The model under review builds one solid part; all positions refer to its coordinate system, in mm. A direction names the side the tool comes from. Give positions to 0.01 mm unless a question says otherwise; leave off trailing zeros. Order: outer loops, then holes, each group sorted by start corner. A loop starts at its lowest first (then second) coordinate and runs counter-clockwise, first axis right, second up. Notation, with made-up numbers: (64.5, 69.25) - (81.5, 69.25) arc R18 ccw to (81.5, 99.25) - close; hole circle Ø2 at (84.25, -23). An arc over 180 degrees is marked (long way). Write item = value, one per line. Start each with the question number.
1. Machinability: for faces 5 (the cylindrical face through (-17, -1, 15)), 6 (the cylindrical face through (-33.56, -29.22, 6.85)), 7 (the cylindrical face through (-17, -15, 24)), 8 (the flat face through (1, -15, -21.822)), 9 (the cylindrical face through (-16.5, -29.22, 15.24)), which of the approach directions +Z, -Z, +X, -X, +Y, -Y give a long, thin tool a straight path to every point of the face, cutting with its end or side? Answer none if there is none.
2. Mouldability with a two-part tool opening along X and no side actions: class faces 1 (the cylindrical face through (16, -15, 23)), 2 (the cylindrical face through (59, -1, 23)), 3 (the flat face through (-100, -15, 0)), 4 (the flat face through (15, -15, 15)) as pulls with the +X half, pulls with the -X half, needs draft (parallel to the pull), parting line crosses it, or undercut.
3. We need section C-C, the plane z = 22.5. Give the boundary of the cut face in (x, y) (3 decimals), and give its area (3 significant figures).
4. We need section B-B, the plane z = -19.5. Give the boundary of the cut face in (x, y).
5. Wall thickness on probe 1 along X at (y, z) = (-16, -12); probe 2 along Y at (x, z) = (32.6, 16.5) (3 decimals); probe 3 along X at (y, z) = (-18, 15.5): over which ranges is each line inside the solid? List them lowest first.
6. We need section A-A, the plane x = 32.6. Give the boundary of the cut face in (y, z) (3 decimals).
7. We need section D-D, the plane y = -21. Give the boundary of the cut face in (x, z), and give its area (3 significant figures).
8. For P1, Ø8, axis at x = -10.5, y = -11, coming from the +Z side, flat-tipped, find the tip position at first contact; note if it passes through.
from build123d import *

# Parameters (mm, degrees)
F1_DEPTH  = 30.65
F2_R      = 5
F3_R      = 5
F4_R      = 5
F5_R      = 5
F6_R      = 5
F7_R      = 5
F8_R      = 5
F9_R      = 5
F10_R     = 3
F11_DEPTH = 20


with BuildPart() as f1:
    # F0 (on Front) → F1 (new body)
    with BuildSketch(Plane.XZ):
        Polygon((-100, 25), (-100, -25), (100, -25), (100, 25), (15, 25), (15, 5.35), (47.5, 5.35), (47.5, -7.066266), (47.5, -21.822188), (0, -21.822188), (-47.5, -21.822188), (-47.5, -7.066266), (-47.5, 5.35), (-15, 5.35), (-15, 25), align=None)
    extrude(amount=F1_DEPTH)

    # F2
    f2_edges = [f1.edges().sort_by_distance(p)[0] for p in [
        (-57.5, -30.65, 25),
    ]]
    fillet(f2_edges, radius=F2_R)

    # F3
    f3_edges = [f1.edges().sort_by_distance(p)[0] for p in [
        (-15, -30.65, 12.675),
    ]]
    fillet(f3_edges, radius=F3_R)

    # F4
    f4_edges = [f1.edges().sort_by_distance(p)[0] for p in [
        (-33.75, -30.65, 5.35),
    ]]
    fillet(f4_edges, radius=F4_R)

    # F5
    f5_edges = [f1.edges().sort_by_distance(p)[0] for p in [
        (15, -30.65, 15.175),
    ]]
    fillet(f5_edges, radius=F5_R)

    # F6
    f6_edges = [f1.edges().sort_by_distance(p)[0] for p in [
        (33.75, -30.65, 5.35),
    ]]
    fillet(f6_edges, radius=F6_R)

    # F7
    f7_edges = [f1.edges().sort_by_distance(p)[0] for p in [
        (60, -30.65, 25),
    ]]
    fillet(f7_edges, radius=F7_R)

    # F8
    f8_edges = [f1.edges().sort_by_distance(p)[0] for p in [
        (60, 0, 25),
    ]]
    fillet(f8_edges, radius=F8_R)

    # F9
    f9_edges = [f1.edges().sort_by_distance(p)[0] for p in [
        (-33.75, 0, 5.35),
    ]]
    fillet(f9_edges, radius=F9_R)

    # F10 (on face) → F11 (cut)
    with BuildSketch(Plane.XY.offset(25)):
        with Locations((-32.6, -15.325)):
            Circle(F10_R)
        with Locations((32.6, -15.325)):
            Circle(F10_R)
    extrude(amount=-F11_DEPTH, mode=Mode.SUBTRACT)


solid = f1.part
Model answer:
q1.face_5 = +Z, +Y
q1.face_6 = -Y
q1.face_7 = +Z, +Y, -Y
q1.face_8 = +Y, -Y
q1.face_9 = +Z, -Y
q2.face_1 = undercut
q2.face_2 = needs draft
q2.face_3 = pulls with the -X half
q2.face_4 = undercut
q3.outline = (-100, -29.98) - (-20, -29.98) arc R4.33 ccw to (-15.67, -25.65) - (-15.67, -5) arc R4.33 ccw to (-20, -0.67) - (-100, -0.67) - close; (15.67, -25.65) arc R4.33 ccw to (20, -29.98) - (100, -29.98) - (100, -0.67) - (20, -0.67) arc R4.33 ccw to (15.67, -5) - close; hole circle Ø6 at (-32.6, -15.325); hole circle Ø6 at (32.6, -15.325)
q3.area = 4,870 mm2
q4.outline = (-100, -30.65) - (-47.5, -30.65) - (-47.5, 0) - (-100, 0) - close; (47.5, -30.65) - (100, -30.65) - (100, 0) - (47.5, 0) - close
q5.probe_1 = -100 to -47.5, 47.5 to 100
q5.probe_2 = -30.65 to -18.325, -12.325 to 0
q5.probe_3 = -100 to -33.96, -31.24 to -15, 15 to 31.24, 33.96 to 100
q6.outline = (-30.65, -25) - (0, -25) - (0, -21.822) - (-30.65, -21.822) - close; (-30.65, 10.35) arc R5 ccw to (-25.65, 5.35) - (-18.325, 5.35) - (-18.325, 25) - (-25.65, 25) arc R5 ccw to (-30.65, 20) - close; (-12.325, 5.35) - (-5, 5.35) arc R5 ccw to (0, 10.35) - (0, 20) arc R5 ccw to (-5, 25) - (-12.325, 25) - close
q7.outline = (-100, -25) - (100, -25) - (100, 25) - (20, 25) arc R5 ccw to (15, 20) - (15, 10.35) arc R5 ccw to (20, 5.35) - (47.5, 5.35) - (47.5, -21.82) - (-47.5, -21.82) - (-47.5, 5.35) - (-20, 5.35) arc R5 ccw to (-15, 10.35) - (-15, 20) arc R5 ccw to (-20, 25) - (-100, 25) - close
q7.area = 6,810 mm2
q8.P1 = -21.82
